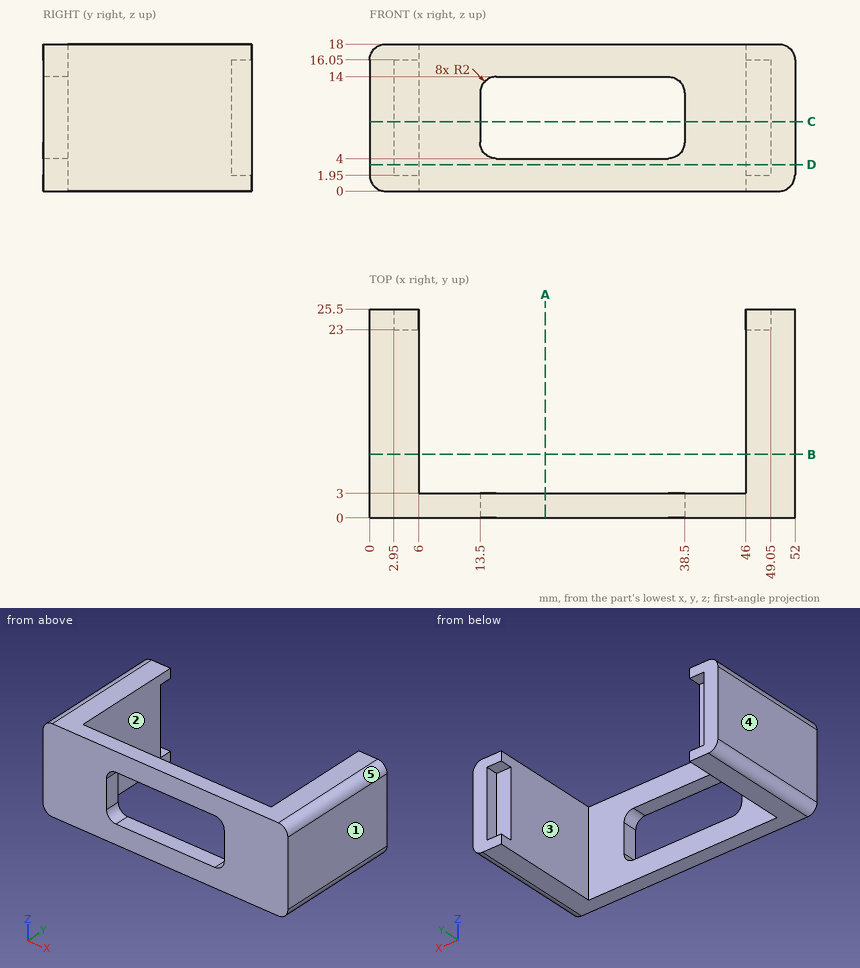
Design review of the part shown in the three views and the two pictorial views. Dimensions are in mm from the part's minimum x, y and z. A direction names the side the tool comes from. Give positions to 0.01 mm unless a question says otherwise; leave off trailing zeros. Loops run counter-clockwise (first coordinate to the right, second up) from the corner with the lowest first, then second, coordinate; pieces in that order, holes last. Notation, with made-up numbers: (74.25, -37.5) -> (116.25, -37.5) arc R16 ccw to (116.25, -10.5) -> close; hole circle Ø10 at (78, -24.75). An arc over 180 degrees is marked (long way). Answer as a JSON object with one key per item and string values. Group by question number.
Q1. Wall thickness on line 1 along X through (y, z) = (15.5, 14); line 2 along X through (y, z) = (2, 7.75); line 3 along Y through (x, z) = (7.5, 14.25): over which ranges is each line inside the solid? List them lowest first.
Q2. Take a section at C-C (z = 8.5). Write out the cut boundary in (x, y).
Q3. Take a section at B-B (y = 7.75). Write out the cut boundary in (x, z), plus the area to 3 significant figures.
Q4. Insertion check: pin 1 (0.8 mm diameter, centred on y = 24.5, z = 7.5, fed in from -X); pin 2 (0.9 mm diameter, centred on x = 48, z = 10.5, fed in from +Y); pin 3 (1.5 mm diameter, centred on x = 43.5, y = 8, fed in from +Z); pin 4 (5.5 mm diameter, centred on x = 19.5, z = 6.5, fed in from +Y). Each pin has a flat end and moves straight along its axis. Give the tip position at first contact, or say it passes through.
Q5. Draft analysis for pull direction X (two halves, no side actions). For the marked faces 3, 4 and 5, state which applies: pulls with the +X half, pulls with the -X half, needs draft (parallel to the pull), parting line crosses it, or undercut.
Q6. Take a section at D-D (z = 3.25). Write out the cut boundary in (x, y).
Q7. Tool access review of the marked faces 1 and 2: name each direction out of +Z, -Z, +X, -X, +Y, -Y from which nothing blocks a thin tool from reaching the whole face with its end or side.
Q8. Take a section at A-A (x = 21.5). Write out the cut boundary in (y, z), plus the area to 3 significant figures.
Answer below:
{
 "1": {"line 1": "x = 0 to 6, 46 to 52", "line 2": "x = 0 to 13.5, 38.5 to 52", "line 3": "y = 0 to 3"},
 "2": {"outline": "(0, 0) -> (13.5, 0) -> (13.5, 3) -> (6, 3) -> (6, 23) -> (2.95, 23) -> (2.95, 25.5) -> (0, 25.5) -> close; (38.5, 0) -> (52, 0) -> (52, 25.5) -> (49.05, 25.5) -> (49.05, 23) -> (46, 23) -> (46, 3) -> (38.5, 3) -> close"},
 "3": {"outline": "(0, 2) arc R2 ccw to (2, 0) -> (6, 0) -> (6, 18) -> (2, 18) arc R2 ccw to (0, 16) -> close; (46, 0) -> (50, 0) arc R2 ccw to (52, 2) -> (52, 16) arc R2 ccw to (50, 18) -> (46, 18) -> close", "area": "213 mm2"},
 "4": {"pin 1": "stops at x = 0", "pin 2": "stops at y = 23", "pin 3": "passes through", "pin 4": "stops at y = 3"},
 "5": {"face 3": "undercut", "face 4": "pulls with the -X half", "face 5": "pulls with the +X half"},
 "6": {"outline": "(0, 0) -> (52, 0) -> (52, 25.5) -> (49.05, 25.5) -> (49.05, 23) -> (46, 23) -> (46, 3) -> (6, 3) -> (6, 23) -> (2.95, 23) -> (2.95, 25.5) -> (0, 25.5) -> close"},
 "7": {"face 1": "+Z, -Z, +X, +Y, -Y", "face 2": "+Z, -Z, +Y"},
 "8": {"outline": "(0, 0) -> (3, 0) -> (3, 4) -> (0, 4) -> close; (0, 14) -> (3, 14) -> (3, 18) -> (0, 18) -> close", "area": "24.0 mm2"}
}
